Could you check a few things on this model? Use its own coordinates, in mm. Face numbers are marked on the shaded views. A direction names the side the tool comes from. Coordinates: 2 decimals unless noted, no trailing zeros. Loops run counter-clockwise (first coordinate to the right, second up) from the corner with the lowest first, then second, coordinate; pieces in that order, holes last. Notation, with made-up numbers: (68.25, 42) - (87.25, 42) arc R19 cw to (87.25, 57) - close; hole circle Ø3 at (4, 55). An arc over 180 degrees is marked (long way). One line per item, written item: value. Start each with the question number.
(1) If we section it at A-A on x = 25: Write out the boundary of the cut face in (y, z) (3 decimals), then the cut area to 3 significant figures.
(2) If I drill on line 1 along Y through (x, z) = (-4.7, 0); line 2 along X through (y, z) = (0.75, 0.25); line 3 along X through (y, z) = (5, 1), over which ranges is the centre line in solid material (lowest first)? Write a range as from..to.
(3) I'm going to push flat-ended pins straight in: P1, Ø6, axis at x = 9, y = 4.5, coming from the -Z side; P2, Ø3, axis at x = 16, y = -1.5, coming from the +Z side (3 decimals); P3, Ø4, axis at y = 1, z = -1, coming from the -X side. Where does each tip first touch, or does it pass through?
(4) If we mould it in two halves opening along Z, with no side actions, what happens to the marked faces 3, 4 and 5? For each: pulls with the +Z half, pulls with the -Z half, needs draft (parallel to the pull), parting line crosses it, or undercut.
(5) On a 3-axis mill with a long thin cutter (end or side, diameter ignored), from which of +Z, -Z, +X, -X, +Y, -Y can I reach the whole of each face in a straight line? I mean the marked faces 1 and 2. Say none if no direction works.
Autodesk Inventor part; units mm, degrees
ref_plane "Work Plane1" through (1.75, 0, 0) normal (0, 0, -1) x (1, 0, 0)
ref_plane "YZ Plane" through (0, 0, 0) normal (1, 0, 0) x (0, 1, 0)
ref_plane "XZ Plane" through (0, 0, 0) normal (0, 1, 0) x (-1, 0, 0)
sketch "Sketch1" plane through (0, 0, 0) normal (0, 0, 1) x (1, 0, 0)
  line L0 (0, 3.175) -> (57.15, 3.175)
  line L1 (57.15, 3.175) -> (57.15, 0)
  line L2 (57.15, 0) -> (0, 0)
  line L3 (0, 0) -> (0, 3.175)
  line L4 (0, -0.635) -> (0, 3.81)
  line L5 (-11.43, 0) -> (68.58, 0)
  dimension "d1" = 6.35
  dimension "d13" = 57.15
revolve "Body" add sketch "Sketch1" angle 360 about axis through (57.15, 0, 0) along (-1, 0, 0)
sketch "Sketch2" plane through (0, 0, 0) normal (-1, 0, 0) x (0, 0, 1)
  line L0 (0, 6.4231) -> (5.5626, 3.2116)
  line L1 (5.5626, 3.2116) -> (5.5626, -3.2116)
  line L2 (5.5626, -3.2116) -> (0, -6.4231)
  line L3 (0, -6.4231) -> (-5.5626, -3.2116)
  line L4 (-5.5626, -3.2116) -> (-5.5626, 3.2116)
  line L5 (-5.5626, 3.2116) -> (0, 6.4231)
  line L6 (-7.7876, 0) -> (7.7876, 0)
  line L7 (0, 8.9924) -> (0, -8.9924)
  point P0 (0, 0)
  point P1 (0, 0)
  point P2 (0, 0)
  dimension "d8" = 11.1252
extrude "Head" add sketch "Sketch2" along normal blind 4.826
sketch "Sketch3" plane through (-4.826, 0, 0) normal (-1, 0, 0) x (0, 0, 1)
  circle A0 centre (0, 0) radius 4.4501
  point P0 (0, 0)
  dimension "d18" = 8.9002
extrude "Indent" cut sketch "Sketch3" against normal blind 0.4836
sketch "Sketch4" plane through (0, 0, 0) normal (0, 0, 1) x (1, 0, 0)
  line L0 (-4.826, 5.5626) -> (-4.826, 6.4231)
  line L1 (-4.826, 6.4231) -> (-4.3292, 6.4231)
  line L2 (-4.3292, 6.4231) -> (-4.826, 5.5626)
  line L3 (-5.7912, 0) -> (0.9652, 0)
  line L4 (0, 6.4231) -> (-4.826, 6.4231)
  line L5 (-4.826, 3.2116) -> (-4.826, 6.4231)
  dimension "d4" = 30
  dimension "d17" = 11.1252
revolve "Chamfer1" cut sketch "Sketch4" angle 360 about axis through (-10, 0, 0) along (1, 0, 0)
thread "Thread"
chamfer "Chamfer2" distance 0.635 distance2 0.6351 1 edges at (57.15, -3.175, 0) measured on face at (57.15, -0.0983, 0.932)
ref_plane "Work Plane1" through (1.75, 0, 0) normal (0, 0, -1) x (1, 0, 0)
equation "\"d1\" = GD"
equation "\"d13\" = NLG"
equation "\"d8\" = SW"
equation "\"d2\" = KOH - SD"
equation "\"d18\" = KOD2"
equation "\"d4\" = ANG1"
equation "\"d17\" = SW"
equation "\"d9\" = GEL"
equation "\"d5\" = -0.5 * SPD + 0.5 * GD"
equation "\"NLG\" = 57.15"
equation "\"GD\" = NND"
equation "\"BDM\" = NND"
equation "\"KOH\" = 4.826"
equation "\"GEL\" = 48.5775"
equation "\"SW\" = 11.1252"
equation "\"SPD\" = GD1"
equation "\"SD\" = 0"
equation "\"ANG1\" = 30deg"
equation "\"GAL\" = 0.635"
equation "\"GUL\" = GAL"
equation "\"KOH2\" = 0.1 * KOH"
equation "\"KOD2\" = 0.8 * SW"
equation "\"GD1\" = 5.08"
equation "\"THREADDIA\" = 6.35"
equation "\"SDH\" = SW"
equation "\"TOA\" = 30deg"
equation "\"RR\" = 0.0635"
equation "\"NND\" = 6.35"
equation "\"SW0\" = SW"
equation "\"SD2\" = NND"
equation "\"E0\" = 1.155 * SW"
properties part number "ANSI B18.6.3 - 1/4-20 UNC - 2.25" material "Steel, Mild"
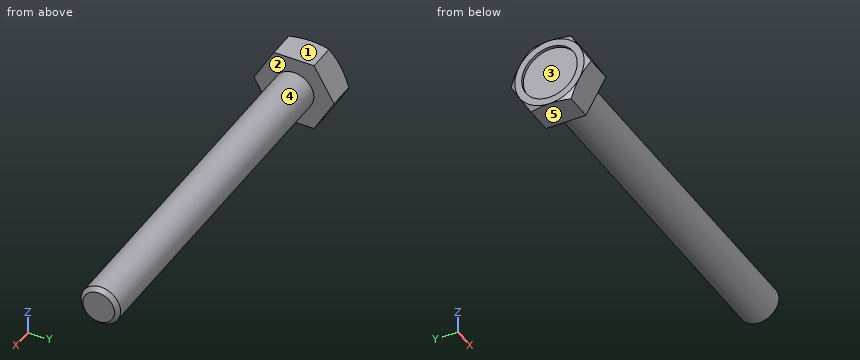
Values:
1. outline: circle Ø6.35 at (0, 0)
1. area: 31.7 mm2
2. line 1: y = -5.78..-4.45, 4.45..5.78
2. line 2: x = -4.34..57.15
2. line 3: x = -4.83..0
3. P1: stops at z = -2.8
3. P2: stops at z = 3.175
3. P3: stops at x = -4.34
4. face 3: undercut
4. face 4: parting line crosses it
4. face 5: pulls with the -Z half
5. face 1: +Z, +X, -X, +Y, -Y
5. face 2: +X
